from build123d import *

# Parameters (mm, degrees)
F1_DEPTH = 25.4
F3_D     = 3.7973
F5_D     = 3.175


with BuildPart() as f1:
    # F0 (on Front) → F1 (new body)
    with BuildSketch(Plane.XZ):
        Polygon((0, 38.1), (0, 0), (38.1, 0), (38.1, 8.636), (33.3375, 8.636), (12.7065850942, 38.1), align=None)
    extrude(amount=-F1_DEPTH)

    # F3 (through all)
    with Locations(Plane.XY.offset(38.1)):
        with Locations((6.3532925471, 19.05), (6.3532925471, 6.35)):
            Hole(F3_D / 2)

    # F5 (through all)
    with Locations(Plane.XZ):
        with Locations((33.3375, 8.636)):
            Hole(F5_D / 2)


solid = f1.part
Geometry: final body of the model. Coordinates: model frame, mm. A direction names the side the tool comes from. Give positions to 0.01 mm unless a question says otherwise; leave off trailing zeros. Write each loop counter-clockwise with the first axis right and the second up, starting at its lowest first coordinate (ties: lowest second). Pieces come first, ordered by that corner, then holes.
(1) Cut plane D-D, the plane x = 36.5. Return loops of the section in (y, z), then the cut area to 3 significant figures.
(2) Ray query, line 1 (Y direction, x = 5, z = 13); line 2 (Y direction, x = 5.5, z = 2); line 3 (X direction, y = 18.25, z = 30.5). Return the intervals inside material, ascending.
(3) Cut plane A-A, the plane y = 19.05. Return loops of the section in (x, z) (1 decimal).
(4) First-contact query: P1, Ø1.6, axis at x = 36, y = 15.5, coming from the +Z side. Flat tip, straight axial feed; report the tip coordinate or a pass-through.
(5) Cut plane C-C, the plane y = 11.25. Return loops of the section in (x, z) (1 decimal).
(6) Cut plane B-B, the plane z = 16. Return loops of the section in (x, y), then the cut area to 3 significant figures.
(7) Access query for faces 1 (the flat face through (38.1, 13, 4)), 2 (the flat face through (37, 13, 8.636)). Directions: +Z, -Z, +X, -X, +Y, -Y. A direction counts if a zero-diameter tool reaches every point of the face in a straight line with its end or side. Return the directions, or none.
(8) Mould query, pull axis Y, two halves, no side actions, for faces 3 (the flat face through (0, 13, 19)), 4 (the cylindrical face through (6.765, 17.196, 18.783)), 5 (the flat face through (15, 25.4, 15)). Classes: released by +Y, released by -Y, zero draft, split by the parting line, or undercut.
Values follow:
1. outline: (0, 0) - (25.4, 0) - (25.4, 8.64) - (0, 8.64) - close
1. area: 219 mm2
2. line 1: y = 0 to 5.02, 7.68 to 17.72, 20.38 to 25.4
2. line 2: y = 0 to 4.65, 8.05 to 17.35, 20.75 to 25.4
2. line 3: x = 0 to 4.63, 8.08 to 18.03
3. outline: (0, 0) - (4.5, 0) - (4.5, 38.1) - (0, 38.1) - close; (8.3, 0) - (38.1, 0) - (38.1, 8.6) - (34.9, 8.6) arc R1.6 cw (long way) to (32.4, 9.9) - (12.7, 38.1) - (8.3, 38.1) - close
4. P1: stops at z = 8.64
5. outline: (0, 0) - (38.1, 0) - (38.1, 8.6) - (34.9, 8.6) arc R1.6 cw (long way) to (32.4, 9.9) - (12.7, 38.1) - (0, 38.1) - close
6. outline: (0, 0) - (28.18, 0) - (28.18, 25.4) - (0, 25.4) - close; hole circle Ø3.8 at (6.35, 6.35); hole circle Ø3.8 at (6.35, 19.05)
6. area: 693 mm2
7. face 1: +Z, -Z, +X, +Y, -Y
7. face 2: +Z, +X, +Y, -Y
8. face 3: zero draft
8. face 4: undercut
8. face 5: released by +Y
